The listing builds one solid part. Answer for the finished solid, in the listing's coordinates (mm). A direction names the side the tool comes from. Give positions to 0.01 mm unless a question says otherwise; leave off trailing zeros. Loops run counter-clockwise (first coordinate to the right, second up) from the corner with the lowest first, then second, coordinate; pieces in that order, holes last. Notation, with made-up numbers: (16.25, 65) - (43.25, 65) arc R32 ccw to (43.25, 94) - close; hole circle Ø5 at (-27.5, -20.5). An arc over 180 degrees is marked (long way). Answer as CSV lines item,"result". Start each with the question number.
1) Flat-ended cylindrical pins translate along their axes: pin 1 (2 mm diameter, centred on x = -1.76, y = 2.38, fed in from +Z); pin 2 (1.3 mm diameter, centred on y = -4.5, z = 2, fed in from +X). Find the tip coordinate at first contact, or state that the pin passes through.
2) A cutting plane is placed at A-A (y = 27.5). Determine the outline of the cut face in (x, z), and give its area (3 significant figures).
3) For faces 1 (the face through (-26, 40.186, 1)), 2 (the face through (7.996, 14, 1)), 3 (the face through (-32.168, -5, 1)), 4 (the face through (3.731, -0.936, 1.479)), determine the directions among +Z, -Z, +X, -X, +Y, -Y from which every point of the face is accessible in a straight line to the end or side of a thin tool.
4) A cutting plane is placed at C-C (y = 19). Determine the outline of the cut face in (x, z), and give its area (3 significant figures).
5) A cutting plane is placed at D-D (y = 1.5). Determine the outline of the cut face in (x, z), and give its area (3 significant figures).
6) For a pull along X with two mould halves and no side action, classify faces 5 (the face through (14.82, 28, 1)), 6 (the face through (-26.455, 3, 1)), 7 (the face through (0.269, 37, 1)), 8 (the face through (-25.55, -4.75, 1.48)) as pulls with the +X half, pulls with the -X half, needs draft (parallel to the pull), parting line crosses it, or undercut.
7) Find the intervals of material crossed by line 1 along X through (y, z) = (38.5, 1.95); line 2 along X through (y, z) = (2.5, 2.7); line 3 along Y through (x, z) = (-22.5, 0.8), in increasing order.
8) A cutting plane is placed at B-B (y = 34). Determine the outline of the cut face in (x, z).
```python
from build123d import *

# Parameters (mm, degrees)
SKETCH2_R           = 1.75
SKETCH2_R_2         = 1.5
SKETCH2_W           = 6.259541377
SKETCH2_H           = 11.363852943
BOSS_EXTRUDE1_DEPTH = 3
SKETCH3_R           = 1.75
BOSS_EXTRUDE2_DEPTH = 3


with BuildPart() as part:
    # Sketch2 → Boss-Extrude1 (new body)
    with BuildSketch(Plane(origin=(0, 0, 0), x_dir=(-1, 0, 0), z_dir=(0, 0, -1))):
        Polygon((-11.441133476, 47.916141751), (-14.819831639, 47.916141751), (-14.819831639, 6.641141751), (-7.995621622, 6.641141751), (-7.995621622, 21.022330273), (-0.780778634, 21.022330273), (-0.780778634, 0.291141751), (26.455168361, 0.291141751), (26.455168361, 5.428807174), (27.667502938, 6.641141751), (39.155168361, 6.641141751), (39.155168361, 47.916141751), (29.679646442, 47.916141751), (29.679646442, 40.185572696), (22.120281557, 40.185572696), (22.120281557, 47.916141751), (-0.269040639, 47.916141751), (-0.269040639, 26.164281213), (-11.441133476, 26.164281213), align=None)
        with Locations((1.761418361, 2.378641751)):
            Circle(SKETCH2_R, mode=Mode.SUBTRACT)
        with Locations((36.067668361, 44.828641751)):
            Circle(SKETCH2_R_2, mode=Mode.SUBTRACT)
        with Locations((22.573918361, 2.378641751)):
            Circle(SKETCH2_R, mode=Mode.SUBTRACT)
        with Locations((-11.732331639, 14.141141751)):
            Circle(SKETCH2_R, mode=Mode.SUBTRACT)
        with Locations((33.207620521, 37.511488804)):
            Rectangle(SKETCH2_W, SKETCH2_H, mode=Mode.SUBTRACT)
    extrude(amount=-BOSS_EXTRUDE1_DEPTH)

    # Sketch3 → Boss-Extrude2 (add)
    # profile 1 of 2: a face of its own
    with BuildSketch(Plane.XY):
        with BuildLine():
            Line((-39.155168361, 47.916141751), (0.269040639, 47.916141751))
            Line((0.269040639, 47.916141751), (0.269040639, 48.797882205))
            Line((0.269040639, 48.797882205), (11.441133476, 48.797882205))
            Line((11.441133476, 48.797882205), (11.441133476, 47.916141751))
            Line((11.441133476, 47.916141751), (14.819831639, 47.916141751))
            Line((14.819831639, 47.916141751), (14.819831639, 50.916141751))
            ThreePointArc((14.819831639, 50.916141751), (13.355365545, 54.451675657), (9.819831639, 55.916141751))
            Line((9.819831639, 55.916141751), (-34.155168361, 55.916141751))
            ThreePointArc((-34.155168361, 55.916141751), (-37.690702267, 54.451675657), (-39.155168361, 50.916141751))
            Line((-39.155168361, 50.916141751), (-39.155168361, 47.916141751))
        make_face()
        with Locations((-27.167668361, 51.416141751)):
            Circle(SKETCH3_R, mode=Mode.SUBTRACT)
        with Locations((2.832331639, 51.416141751)):
            Circle(SKETCH3_R, mode=Mode.SUBTRACT)
    # profile 2 of 2: a face of its own
    with BuildSketch(Plane.XY):
        with BuildLine():
            Line((-26.455168361, 0.291141751), (-31.080954927, -2.083201693))
            ThreePointArc((-31.080954927, -2.083201693), (-31.87450361, -2.820045974), (-32.167668361, -3.862501457))
            Line((-32.167668361, -3.862501457), (-32.167668361, -5.640994596))
            ThreePointArc((-32.167668361, -5.640994596), (-31.581881924, -7.055208159), (-30.167668361, -7.640994596))
            Line((-30.167668361, -7.640994596), (5.832331639, -7.640994596))
            ThreePointArc((5.832331639, -7.640994596), (7.246545201, -7.055208159), (7.832331639, -5.640994596))
            Line((7.832331639, -5.640994596), (7.832331639, -3.975377608))
            ThreePointArc((7.832331639, -3.975377608), (7.496029114, -2.865372784), (6.600220929, -2.128665384))
            Line((6.600220929, -2.128665384), (0.780778634, 0.291141751))
            Line((0.780778634, 0.291141751), (-26.455168361, 0.291141751))
        make_face()
        with Locations((-27.167668361, -4.083858249)):
            Circle(SKETCH3_R, mode=Mode.SUBTRACT)
        with Locations((2.832331639, -4.083858249)):
            Circle(SKETCH3_R, mode=Mode.SUBTRACT)
    extrude(amount=BOSS_EXTRUDE2_DEPTH)


solid = part.part
```
Ans:
1,pin 1,"through"
1,pin 2,"x = 7.83"
2,outline,"(-39.16, 0) - (0.27, 0) - (0.27, 3) - (-39.16, 3) - close; (11.44, 0) - (14.82, 0) - (14.82, 3) - (11.44, 3) - close"
2,area,"128 mm2"
3,face 1,"+Z, -Z"
3,face 2,"+Z, -Z, -Y"
3,face 3,"+Z, -Z, -X, -Y"
3,face 4,"+Z, -Z, +X"
4,outline,"(-39.16, 0) - (0.78, 0) - (0.78, 3) - (-39.16, 3) - close; (8, 0) - (14.82, 0) - (14.82, 3) - (8, 3) - close"
4,area,"140 mm2"
5,outline,"(-26.46, 0) - (-24.09, 0) - (-24.09, 3) - (-26.46, 3) - close; (-21.06, 0) - (-3.27, 0) - (-3.27, 3) - (-21.06, 3) - close; (-0.25, 0) - (0.78, 0) - (0.78, 3) - (-0.25, 3) - close"
5,area,"63.5 mm2"
6,face 5,"pulls with the +X half"
6,face 6,"pulls with the -X half"
6,face 7,"undercut"
6,face 8,"undercut"
7,line 1,"-39.16 to -36.34, -30.08 to 0.27, 11.44 to 14.82"
7,line 2,"-26.46 to -24.32, -20.83 to -3.51, -0.02 to 0.78"
7,line 3,"-7.64 to 0.63, 4.13 to 40.19, 47.92 to 55.92"
8,outline,"(-39.16, 0) - (-36.34, 0) - (-36.34, 3) - (-39.16, 3) - close; (-30.08, 0) - (0.27, 0) - (0.27, 3) - (-30.08, 3) - close; (11.44, 0) - (14.82, 0) - (14.82, 3) - (11.44, 3) - close"
